Work out the finished part from the listing and answer in its coordinate system (mm). A direction names the side the tool comes from. Coordinates: 2 decimals unless noted, no trailing zeros. Order: outer loops, then holes, each group sorted by start corner. A loop starts at its lowest first (then second) coordinate and runs counter-clockwise, first axis right, second up. Notation, with made-up numbers: (29, 2.5) - (73, 2.5) arc R12 ccw to (73, 7.5) - close; hole circle Ø8 at (56, -24). An arc over 180 degrees is marked (long way). Answer as a JSON object with one key per item and string values. Group by question number.
1) Section B-B (z = 23.5) is taken. Give the vertices of the cut face in (x, y), plus the area to 3 significant figures.
2) Section A-A (x = 46) is taken. Give the vertices of the cut face in (y, z).
3) Section C-C (y = 30.5) is taken. Give the vertices of the cut face in (x, z), plus the area to 3 significant figures.
4) Each of these flat-tipped pins is pushed along its axis until it touches: P1, Ø24.5, axis at x = 27, y = 15, coming from the +Z side; P2, Ø12, axis at y = 41.5, z = 34.5, coming from the +X side; P3, Ø10, axis at x = 42, z = 28.5, coming from the +Y side. Where does it stop, or does it pass through?
5) Section D-D (x = 26.5) is taken. Give the vertices of the cut face in (y, z).
6) A tool of negligible diameter and unlimited length cuts with its end or side. For faces 1 (the face through (24, 22, 20)), 2 (the face through (-1.303, 5.532, 32.395)), from which of +Z, -Z, +X, -X, +Y, -Y can it reach the whole face along a straight path? Write none if from no direction.
7) Find the intervals of material crossed by line 1 along Z through (x, y) = (25.5, 20.5); line 2 along Y through (x, z) = (13.5, 22) (3 decimals); line 3 along Y through (x, z) = (2.5, 26.75), in increasing order.
8) The mould has two halves that part along X. Classify faces 3 (the face through (27.03, 19.7, 22.46)), 4 (the face through (24, 22, 25)), 5 (the face through (43.237, 40.239, 22.535)), 6 (the face through (19.925, 26.788, 22.465)): released by +X, released by -X, zero draft, split by the parting line, or undercut.
from build123d import *

# Parameters (mm, degrees)
F0_W      = 140
F0_H      = 120
F1_DEPTH  = 25
F2_R      = 4.15
F3_DEPTH  = 25.001
F4_R      = 2.5
F5_DEPTH  = 25
F7_DEPTH  = 50.001
F9_DEPTH  = 20
F10_R     = 2.5
F10_R_2   = 2
F11_DEPTH = 10


with BuildPart() as f1:
    # F0 (on Top) → F1 (new body)
    with BuildSketch(Plane.XY):
        Rectangle(F0_W, F0_H)
    extrude(amount=F1_DEPTH)

    # F2 (on face) → F3 (cut, through all)
    with BuildSketch(Plane.XY.offset(25)):
        with Locations((46.530288, 42.764347)):
            Circle(F2_R)
    extrude(amount=-F3_DEPTH, mode=Mode.SUBTRACT)

    # F4 (on face) → F5 (join)
    with BuildSketch(Plane.XY.offset(25)):
        with Locations((0.539839, 3.842103)):
            Circle(F4_R)
    extrude(amount=F5_DEPTH)

    # F6 (on face) → F7 (intersect, through all)
    with BuildSketch(Plane(origin=(0, 0, 0), x_dir=(1, 0, 0), z_dir=(0, 0, -1))):
        with BuildLine():
            Line((-2.423829, -7.228351), (42.908028, -46.903095))
            ThreePointArc((42.908028, -46.903095), (50.728586, -46.317415), (50.013185, -38.507655))
            Line((50.013185, -38.507655), (3.389482, -0.359355))
            ThreePointArc((3.389482, -0.359355), (-2.895133, -0.935047), (-2.423829, -7.228351))
        make_face()
    extrude(amount=-F7_DEPTH, mode=Mode.INTERSECT)

    # F8 (on face) → F9 (cut)
    with BuildSketch(Plane(origin=(0, 0, 0), x_dir=(1, 0, 0), z_dir=(0, 0, -1))):
        with BuildLine():
            ThreePointArc((42.908028, -46.903095), (50.728586, -46.317415), (50.013185, -38.507655))
            Line((50.013185, -38.507655), (3.389482, -0.359355))
            ThreePointArc((3.389482, -0.359355), (-2.895133, -0.935047), (-2.423829, -7.228351))
            Line((-2.423829, -7.228351), (42.908028, -46.903095))
        make_face()
    extrude(amount=-F9_DEPTH, mode=Mode.SUBTRACT)

    # F10 (on face) → F11 (cut)
    with BuildSketch(Plane.XY.offset(50)):
        with Locations((0.539839, 3.842103)):
            Circle(F10_R)
        with Locations((0.539839, 3.842103)):
            Circle(F10_R_2, mode=Mode.SUBTRACT)
    extrude(amount=-F11_DEPTH, mode=Mode.SUBTRACT)


solid = f1.part
Report:
{
 "1": {"outline": "(-2.42, 7.23) arc R4.5 ccw to (3.39, 0.36) - (50.01, 38.51) arc R5.5 ccw (long way) to (42.91, 46.9) - close; hole circle Ø8.3 at (46.53, 42.76)", "area": "628 mm²"},
 "2": {"outline": "(35.22, 20) - (38.65, 20) - (38.65, 25) - (35.22, 25) - close; (46.88, 20) - (48.24, 20) - (48.24, 25) - (46.88, 25) - close"},
 "3": {"outline": "(24.17, 20) - (40.23, 20) - (40.23, 25) - (24.17, 25) - close", "area": "80.3 mm²"},
 "4": {"P1": "stops at z = 25", "P2": "passes through", "P3": "stops at y = 48.18"},
 "5": {"outline": "(19.27, 20) - (32.54, 20) - (32.54, 25) - (19.27, 25) - close"},
 "6": {"face 1": "-Z, +X, -X, +Y, -Y", "face 2": "+Z"},
 "7": {"line 1": "z = 20 to 25", "line 2": "y = 8.632 to 21.165", "line 3": "y = 2.29 to 5.39"},
 "8": {"face 3": "released by +X", "face 4": "zero draft", "face 5": "undercut", "face 6": "released by -X"}
}
